Check sheet for the modelled part. Datum: model origin and axes. Units: mm. A direction names the side the tool comes from. Coordinates: 2 decimals unless noted, no trailing zeros. Loops run counter-clockwise (first coordinate to the right, second up) from the corner with the lowest first, then second, coordinate; pieces in that order, holes last. Notation, with made-up numbers: (51.5, 75.5) - (67.5, 75.5) arc R25 ccw to (67.5, 89.5) - close; hole circle Ø8 at (-32, 67.25). An arc over 180 degrees is marked (long way). Use a Markdown table: item, result. Add a question column.
1) Thickness scan on line 1 (Y direction, x = 8.5, z = 77); line 2 (Y direction, x = 11, z = 45.5); line 3 (X direction, y = 22, z = 28.5). Record the ranges inside material, lowest first.
2) Go/stop test with flat-tipped pins: P1, Ø5, axis at y = 43.5, z = 14, coming from the +X side; P2, Ø1, axis at y = -37, z = 69, coming from the +X side; P3, Ø2, axis at y = 13.5, z = 31.5, coming from the -X side. Record where each tip stops, or that it passes through.
3) Sectioned sample at B-B, the plane y = 0. Enter the section's corners in (x, z).
4) Sectioned sample at C-C, the plane z = 88.5. Enter the section's corners in (x, y).
5) Sectioned sample at A-A, the plane x = 0. Enter the section's corners in (y, z), then the cut area to 3 significant figures.
6) Draft check along Y on faces 5 (the flat face through (-1, -12, 97.79)), 6 (the cylindrical face through (-13.77, -61.99, 48.28)), 7 (the flat face through (-20.632, 7.072, 95.858)). Enter one of: pulls with the +Y half, pulls with the -Y half, needs draft (parallel to the pull), parting line crosses it, or undercut.
7) Tool access check on faces 1 (the flat face through (16.036, 7, 50)), 2 (the flat face through (-1, -12, 0)), 3 (the flat face through (-1.66, -9.76, 1.93)), 4 (the flat face through (17.914, 7.072, 95.858)). Record the directions out of +Z, -Z, +X, -X, +Y, -Y that give a thin tool (end or side, any length) a straight path to the whole face; none if there is none.
from build123d import *

# Parameters (mm, degrees)
F0_R     = 63.5
F1_DEPTH = 97.79
F2_W     = 34.789767
F2_H     = 30.441041
F3_DEPTH = 97.791
F4_R     = 5.08
F5_SIZE  = 3.81


with BuildPart() as f1:
    # F0 (on Top) → F1 (new body)
    with BuildSketch(Plane.XY):
        Circle(F0_R)
    extrude(amount=F1_DEPTH)

    # F2 (on face) → F3 (cut, through all)
    with BuildSketch(Plane.XY.offset(97.79)):
        with Locations((-1.358978, 7.338465)):
            Rectangle(F2_W, F2_H)
    extrude(amount=-F3_DEPTH, mode=Mode.SUBTRACT)

    # F4
    f4_edges = [f1.edges().sort_by_distance(p)[0] for p in [
        (-63.5, 0, 97.79),
        (-63.5, 0, 0),
    ]]
    fillet(f4_edges, radius=F4_R)

    # F5
    f5_edges = [f1.edges().sort_by_distance(p)[0] for p in [
        (-1.358978, -7.882056, 0),
        (16.035905, 7.338465, 0),
        (-1.358978, 22.558985, 0),
        (-18.753862, 7.338465, 0),
        (16.035905, 7.338465, 97.79),
        (-1.358978, 22.558985, 97.79),
        (-18.753862, 7.338465, 97.79),
        (-1.358978, -7.882056, 97.79),
    ]]
    chamfer(f5_edges, length=F5_SIZE)


solid = f1.part
Solved:
| question | item | result |
|---|---|---|
| 1 | line 1 | y = -62.93 to -7.88, 22.56 to 62.93 |
| 1 | line 2 | y = -62.54 to -7.88, 22.56 to 62.54 |
| 1 | line 3 | x = -59.57 to -18.75, 16.04 to 59.57 |
| 2 | P1 | stops at x = 48.49 |
| 2 | P2 | stops at x = 51.96 |
| 2 | P3 | stops at x = -62.26 |
| 3 | outline | (-63.5, 5.08) arc R5.08 ccw to (-58.42, 0) - (-22.56, 0) - (-18.75, 3.81) - (-18.75, 93.98) - (-22.56, 97.79) - (-58.42, 97.79) arc R5.08 ccw to (-63.5, 92.71) - close; (16.04, 3.81) - (19.85, 0) - (58.42, 0) arc R5.08 ccw to (63.5, 5.08) - (63.5, 92.71) arc R5.08 ccw to (58.42, 97.79) - (19.85, 97.79) - (16.04, 93.98) - close |
| 4 | outline | circle Ø127 at (0, 0); hole (-18.75, -7.88) - (16.04, -7.88) - (16.04, 22.56) - (-18.75, 22.56) - close |
| 5 | outline | (-63.5, 5.08) arc R5.08 ccw to (-58.42, 0) - (-11.69, 0) - (-7.88, 3.81) - (-7.88, 93.98) - (-11.69, 97.79) - (-58.42, 97.79) arc R5.08 ccw to (-63.5, 92.71) - close; (22.56, 3.81) - (26.37, 0) - (58.42, 0) arc R5.08 ccw to (63.5, 5.08) - (63.5, 92.71) arc R5.08 ccw to (58.42, 97.79) - (26.37, 97.79) - (22.56, 93.98) - close |
| 5 | area | 9,390 mm2 |
| 6 | face 5 | needs draft |
| 6 | face 6 | parting line crosses it |
| 6 | face 7 | undercut |
| 7 | face 1 | +Z, -Z |
| 7 | face 2 | -Z, +X, -X, +Y, -Y |
| 7 | face 3 | -Z |
| 7 | face 4 | +Z |
